Input: dimensioned drawing with shaded views. Units: mm. Origin: part minimum x, y, z. A direction names the side the tool comes from. Round coordinates to 2 decimals unless told otherwise and drop trailing zeros. Loops run counter-clockwise (first coordinate to the right, second up) from the corner with the lowest first, then second, coordinate; pieces in that order, holes last. Notation, with made-up numbers: M 17.25,56.25 L 30.25,56.25 A21 cw 30.25,67.25 Z; hole C 36.25,2 d9. An arc over 180 degrees is marked long. Return JSON: item names as keys, results as strings.
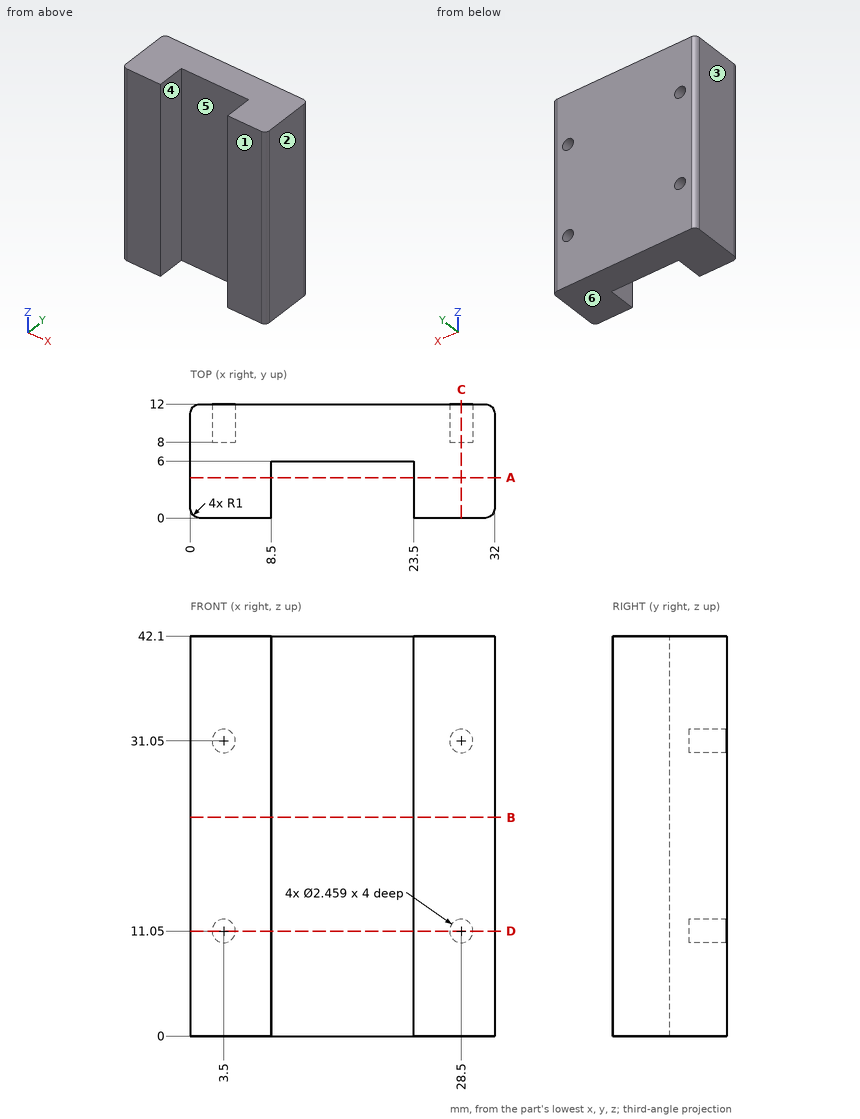
Q1. Section query D-D (z = 11.05). Output: boundary loops of the cut face in (x, y), plus the area to 3 significant figures.
Determined:
{"outline": "M 0,1 A1 ccw 1,0 L 8.5,0 L 8.5,6 L 23.5,6 L 23.5,0 L 31,0 A1 ccw 32,1 L 32,11 A1 ccw 31,12 L 29.73,12 L 29.73,8 L 27.27,8 L 27.27,12 L 4.73,12 L 4.73,8 L 2.27,8 L 2.27,12 L 1,12 A1 ccw 0,11 Z", "area": "273 mm^2"}
Q2. Pull-direction query (X, two-part tool) for the marked faces 1, 2, 3 and 4; classes: pulls with the +X half, pulls with the -X half, needs draft (parallel to the pull), parting line crosses it, or undercut.
Determined:
{"face 1": "needs draft", "face 2": "pulls with the +X half", "face 3": "pulls with the -X half", "face 4": "undercut"}
Q3. Reachability of the marked faces 5 and 6 from +Z, -Z, +X, -X, +Y, -Y: full face, straight path, thin tool, end or side. Return the list, or none.
Determined:
{"face 5": "+Z, -Z, -Y", "face 6": "-Z, +X, -X, +Y, -Y"}
Q4. Material intervals for L1, parallel to Z at x = 3.5, y = 10.45; L2, parallel to X at y = 10.65, z = 11.05; L3, parallel to X at y = 3, z = 19, sorted ascending.
Determined:
{"L1": "z = 0 to 9.82, 12.28 to 29.82, 32.28 to 42.1", "L2": "x = 0 to 2.27, 4.73 to 27.27, 29.73 to 32", "L3": "x = 0 to 8.5, 23.5 to 32"}
Q5. Section query C-C (x = 28.5). Output: boundary loops of the cut face in (y, z), plus the area to 3 significant figures.
Determined:
{"outline": "M 0,0 L 12,0 L 12,9.82 L 8,9.82 L 8,12.28 L 12,12.28 L 12,29.82 L 8,29.82 L 8,32.28 L 12,32.28 L 12,42.1 L 0,42.1 Z", "area": "486 mm^2"}
Q6. Section query B-B (z = 23). Output: boundary loops of the cut face in (x, y), plus the area to 3 significant figures.
Determined:
{"outline": "M 0,1 A1 ccw 1,0 L 8.5,0 L 8.5,6 L 23.5,6 L 23.5,0 L 31,0 A1 ccw 32,1 L 32,11 A1 ccw 31,12 L 1,12 A1 ccw 0,11 Z", "area": "293 mm^2"}
Q7. Pin query (flat end, axial travel): pin 1 (1.2 mm diameter, centred on x = 3.5, z = 31.5, fed in from +Y); pin 2 (7.5 mm diameter, centred on x = 15.5, z = 18, fed in from -Y). Return the tip coordinate at first contact, or that it passes through.
Determined:
{"pin 1": "stops at y = 8", "pin 2": "stops at y = 6"}
Q8. Section query A-A (y = 4.25). Output: boundary loops of the cut face in (x, z), plus the area to 3 significant figures.
Determined:
{"outline": "M 0,0 L 8.5,0 L 8.5,42.1 L 0,42.1 Z; M 23.5,0 L 32,0 L 32,42.1 L 23.5,42.1 Z", "area": "716 mm^2"}
